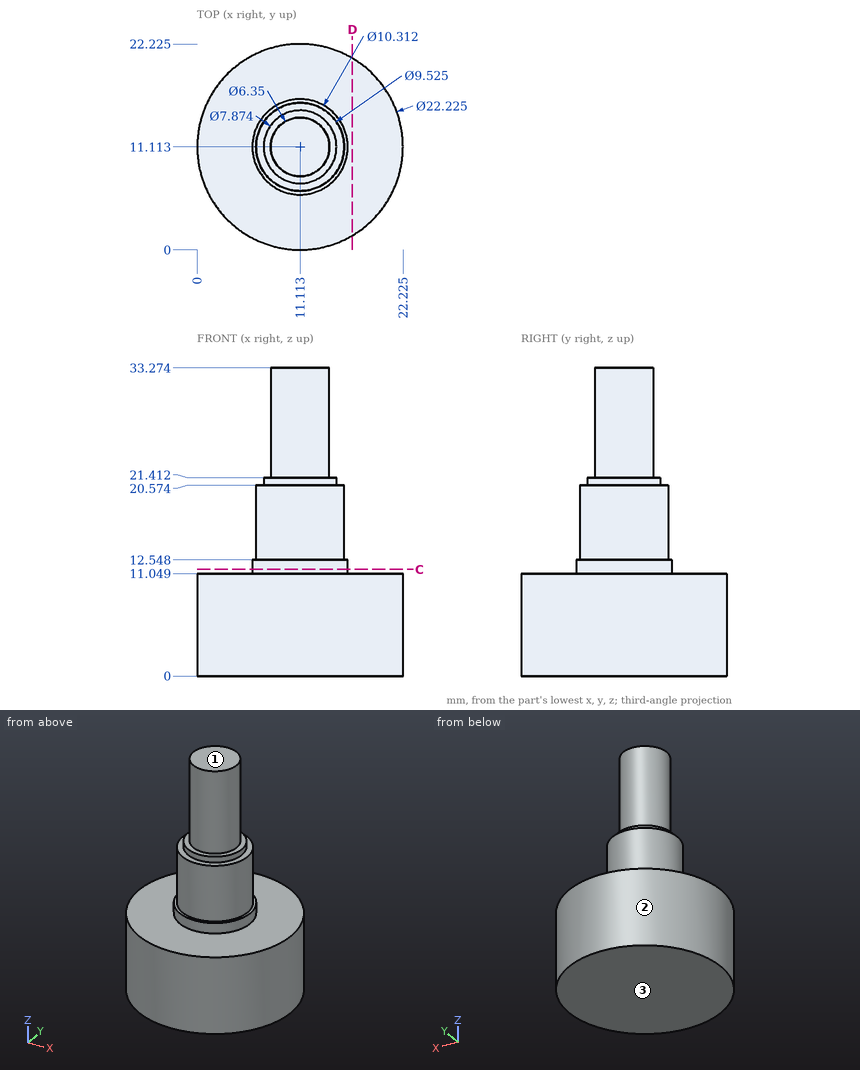
The drawing under review shows one solid part. Ordinate dimensions are in mm from its lowest x, y, z. Round coordinates to 2 decimals unless told otherwise and drop trailing zeros. Order: outer loops, then holes, each group sorted by start corner. A loop starts at its lowest first (then second) coordinate and runs counter-clockwise, first axis right, second up. Notation, with made-up numbers: M -36.75,-32.75 L -0.75,-32.75 A13 ccw -0.75,-24.75 Z; hole C 87.5,15 d2. An arc over 180 degrees is marked long. Answer as CSV lines item,"result". Start each with the question number.
1) The part is to be moulded in two halves that separate along Z. For the marked faces 1, 2 and 3, say which applies: +Z half, -Z half, draft (parallel to the pull), parting line (faces both ways), or undercut.
2) Add section C-C (z = 11.5). Give the boundary of the cut face in (x, y).
3) For pin 1 Ø1.5 at (x, y) = (8.5, 12.5) entering from -Z; pin 2 Ø1.5 at (y, z) = (16.5, 5) entering from -X (1 decimal); pin 3 Ø1.5 at (x, y) = (14, 19.5) entering from +Z; pin 4 Ø4 at (y, z) = (4, 5) entering from -X (1 decimal), all flat-tipped, find the tip position at first contact; note any pin that passes through.
4) Add section D-D (x = 16.75). Give the boundary of the cut face in (y, z).
5) Wall thickness on line 1 along Z through (x, y) = (7.5, 17.75); line 2 along Z through (x, y) = (15.25, 9) (1 decimal); line 3 along X through (y, z) = (11, 31) (1 decimal): over which ranges is each line inside the solid? List them lowest first. Write a range as [from, to].
Resolved:
1,face 1,"+Z half"
1,face 2,"draft"
1,face 3,"-Z half"
2,outline,"C 11.11,11.11 d10.31"
3,pin 1,"z = 0"
3,pin 2,"x = 1"
3,pin 3,"z = 11.05"
3,pin 4,"x = 1.2"
4,outline,"M 1.54,0 L 20.69,0 L 20.69,11.05 L 1.54,11.05 Z"
5,line 1,"[0, 11.05]"
5,line 2,"[0, 20.6]"
5,line 3,"[7.9, 14.3]"
